```python
from build123d import *

# Parameters (mm, degrees)
SKETCH_2_W                       = 64.02174429
SKETCH_2_H                       = 9.248919907
CUT_EXTRUDE_1_DEPTH              = 49
HOLE_WIZARD_M4_2_D               = 3.3
HOLE_WIZARD_M4_2_DEPTH           = 5.5
HOLE_WIZARD_M4_2_TIP             = 0.991420021
HOLE_WIZARD_M6_2_D               = 5
HOLE_WIZARD_M6_2_DEPTH           = 5.5
HOLE_WIZARD_M6_2_TIP             = 1.502151548
HOLE_WIZARD_M4_3_D               = 3.3
HOLE_WIZARD_M4_3_DEPTH           = 13.4
HOLE_WIZARD_M4_3_TIP             = 0.991420021
HOLE_WIZARD_M4_3_ON_FACE_2_D     = 3.3
HOLE_WIZARD_M4_3_ON_FACE_2_DEPTH = 13.4
HOLE_WIZARD_M4_3_ON_FACE_2_TIP   = 0.991420021


with BuildPart() as part:
    # 草图1 → 旋转1 (revolve)
    with BuildSketch(Plane(origin=(0, 0, 0), x_dir=(1, 0, 0), z_dir=(0, 1, 0)), mode=Mode.PRIVATE) as revolve_1_sk:
        Polygon((28.5, 7.5), (28.5, -7.5), (19.05, -7.5), (19.05, -4), (20.15, -4), (20.15, 4), (19.05, 4), (19.05, 7.5), align=None)
    revolve(revolve_1_sk.sketch.rotate(Axis((0, 0, -31.9390681), (0, 0, 1)), 180), axis=Axis((0, 0, -31.9390681), (0, 0, 1)))  # turned: the seam where the file's is

    # 草图2 → 切除-拉伸1 (cut)
    with BuildSketch(Plane.XY.offset(7.5)):
        with Locations((-1.141100508, 32.324459954)):
            Rectangle(SKETCH_2_W, SKETCH_2_H)
        with Locations((-1.141100508, -32.324459954)):
            Rectangle(SKETCH_2_W, SKETCH_2_H)
    extrude(amount=-CUT_EXTRUDE_1_DEPTH, mode=Mode.SUBTRACT)

    # M4 螺纹孔2
    with Locations(Plane(origin=(0, 27.7, 0), x_dir=(1, 0, 0), z_dir=(0, 1, 0))):
        with Locations((0, 0)):
            Hole(HOLE_WIZARD_M4_2_D / 2, depth=HOLE_WIZARD_M4_2_DEPTH)
            with Locations((0, 0, -(HOLE_WIZARD_M4_2_DEPTH + HOLE_WIZARD_M4_2_TIP / 2))):  # 118° drill point
                Cone(0, HOLE_WIZARD_M4_2_D / 2, HOLE_WIZARD_M4_2_TIP, mode=Mode.SUBTRACT)

    # M6 螺纹孔2
    with Locations(Plane(origin=(0, -27.7, 0), x_dir=(-1, 0, 0), z_dir=(0, -1, 0))):
        with Locations((0, 0)):
            Hole(HOLE_WIZARD_M6_2_D / 2, depth=HOLE_WIZARD_M6_2_DEPTH)
            with Locations((0, 0, -(HOLE_WIZARD_M6_2_DEPTH + HOLE_WIZARD_M6_2_TIP / 2))):  # 118° drill point
                Cone(0, HOLE_WIZARD_M6_2_D / 2, HOLE_WIZARD_M6_2_TIP, mode=Mode.SUBTRACT)

    # M4 螺纹孔3
    with Locations(Plane(origin=(24.681724008, 14.25, 0), x_dir=(-0.5, 0.866025404, 0), z_dir=(0.866025404, 0.5, 0))):
        with Locations((0, 0)):
            Hole(HOLE_WIZARD_M4_3_D / 2, depth=HOLE_WIZARD_M4_3_DEPTH)
            with Locations((0, 0, -(HOLE_WIZARD_M4_3_DEPTH + HOLE_WIZARD_M4_3_TIP / 2))):  # 118° drill point
                Cone(0, HOLE_WIZARD_M4_3_D / 2, HOLE_WIZARD_M4_3_TIP, mode=Mode.SUBTRACT)

    # M4 螺纹孔3 on face 2
    with Locations(Plane(origin=(-24.681724008, 14.25, 0), x_dir=(-0.500000175, -0.866025303, 0), z_dir=(-0.866025303, 0.500000175, 0))):
        with Locations((0, 0)):
            Hole(HOLE_WIZARD_M4_3_ON_FACE_2_D / 2, depth=HOLE_WIZARD_M4_3_ON_FACE_2_DEPTH)
            with Locations((0, 0, -(HOLE_WIZARD_M4_3_ON_FACE_2_DEPTH + HOLE_WIZARD_M4_3_ON_FACE_2_TIP / 2))):  # 118° drill point
                Cone(0, HOLE_WIZARD_M4_3_ON_FACE_2_D / 2, HOLE_WIZARD_M4_3_ON_FACE_2_TIP, mode=Mode.SUBTRACT)


solid = part.part
```
Build history of the part. All positions in model axes, mm. A direction names the side the tool comes from. Give positions to 0.01 mm unless a question says otherwise; leave off trailing zeros. Loops run counter-clockwise (first coordinate to the right, second up) from the corner with the lowest first, then second, coordinate; pieces in that order, holes last. Notation, with made-up numbers: (-31, -33.5) - (-1, -33.5) arc R30 ccw to (-1, 1.5) - close; hole circle Ø5 at (30, 73.25). An arc over 180 degrees is marked (long way). Use a Markdown table: item, result.
(1) Band-saw the part on B-B (y = 4). Give the cut face in (x, z), and give its area (3 significant figures).
Taken from the geometry:
| item | result |
|---|---|
| outline | (-28.22, -7.5) - (-18.63, -7.5) - (-18.63, -4) - (-19.75, -4) - (-19.75, 4) - (-18.63, 4) - (-18.63, 7.5) - (-28.22, 7.5) - close; (18.63, -7.5) - (28.22, -7.5) - (28.22, 7.5) - (18.63, 7.5) - (18.63, 4) - (19.75, 4) - (19.75, -4) - (18.63, -4) - close |
| area | 270 mm2 |
(2) Band-saw the part on A-A (x = -14). Give the cut face in (y, z).
Taken from the geometry:
| item | result |
|---|---|
| outline | (-24.82, -7.5) - (-12.92, -7.5) - (-12.92, -4) - (-14.49, -4) - (-14.49, 4) - (-12.92, 4) - (-12.92, 7.5) - (-24.82, 7.5) - close; (12.92, -7.5) - (24.82, -7.5) - (24.82, 7.5) - (12.92, 7.5) - (12.92, 4) - (14.49, 4) - (14.49, -4) - (12.92, -4) - close |
(3) Pull direction X, two halves, no side cores. Call faces 4 (the face through (28.495, -0.532, 0.105)), 5 (the face through (-0.54, -24.91, 2.44)), 6 (the face through (19.4, -0.4, 7.5)): +X half, -X half, draft (parallel to the pull), parting line (faces both ways), or undercut.
Taken from the geometry:
| item | result |
|---|---|
| face 4 | +X half |
| face 5 | undercut |
| face 6 | draft |
(4) Drop flat-ended pins along their axis: pin 1 Ø10 at (x, y) = (10.5, -5.5) entering from -Z; pin 2 Ø1.5 at (y, z) = (-2.5, 6) entering from -X; pin 3 Ø3 at (x, z) = (-9, -3) entering from +Y; pin 4 Ø3 at (x, z) = (0, 0) entering from -Y. Give the stop position or say it passes through.
Taken from the geometry:
| item | result |
|---|---|
| pin 1 | through |
| pin 2 | x = -28.45 |
| pin 3 | y = 27.5 |
| pin 4 | y = -21.6 |
(5) Wall check: line 1 along Z through (x, y) = (0, 24); line 2 along Y through (x, z) = (0, -5.85); line 3 along Y through (x, z) = (13, -6). Give the ranges that are in metal, low to high.
Taken from the geometry:
| item | result |
|---|---|
| line 1 | -7.5 to -1.65, 1.65 to 7.5 |
| line 2 | -27.7 to -19.05, 19.05 to 27.7 |
| line 3 | -25.36 to -13.92, 13.92 to 25.36 |
(6) Which spindle directions (+Z, -Z, +X, -X, +Y, -Y) get a long thin tool onto all of the face, cutting with end or side? Do faces 1 (the face through (-12, 15, 4)), 2 (the face through (4.13, 18.597, -5.774)), 3 (the face through (1.216, 24.912, -1.115)). Say none if no direction does.
Taken from the geometry:
| item | result |
|---|---|
| face 1 | none |
| face 2 | +Z, -Z |
| face 3 | +Y |
